The model under review builds one solid part; all positions refer to its coordinate system, in mm. A direction names the side the tool comes from. Coordinates: 2 decimals unless noted, no trailing zeros. Write each loop counter-clockwise with the first axis right and the second up, starting at its lowest first coordinate (ties: lowest second). Pieces come first, ordered by that corner, then holes. Notation, with made-up numbers: M 25,42 L 76,42 A10 cw 76,55 Z; hole C 33,78.5 d4. An arc over 180 degrees is marked long. Answer as CSV lines item,"result". Start each with the question number.
Autodesk Fusion 360 part; units mm, degrees
sketch "Skizze1" plane through (0, 0, 0) normal (0, 0, 1) x (1, 0, 0)
  line L0 (12.8, 3.8) -> (-12.8, 3.8)
  line L1 (-12.8, 3.8) -> (-12.8, -3.8)
  line L2 (-12.8, -3.8) -> (12.8, -3.8)
  line L3 (12.8, -3.8) -> (12.8, 3.8)
  line L4 (12.8, 3.8) -> (-12.8, -3.8) construction
  line L5 (-12.8, 3.8) -> (12.8, -3.8) construction
  line L6 (-15.6, 6.6) -> (-15.6, -6.6)
  line L7 (-15.6, -6.6) -> (15.6, -6.6)
  line L8 (15.6, -6.6) -> (15.6, 6.6)
  line L9 (15.6, 6.6) -> (-15.6, 6.6)
  line L10 (12.8, 1.5) -> (-12.8, 1.5)
  line L11 (-12.8, 1.5) -> (-12.8, -1.5)
  line L12 (-12.8, -1.5) -> (12.8, -1.5)
  line L13 (12.8, -1.5) -> (12.8, 1.5)
  line L14 (12.8, 1.5) -> (-12.8, -1.5) construction
  line L15 (-12.8, 1.5) -> (12.8, -1.5) construction
  circle A0 centre (20.6, 0) radius 1.6
  circle A1 centre (-20.6, 0) radius 1.6
  circle A2 centre (20.6, 0) radius 4
  circle A3 centre (-20.6, 0) radius 4
  line L16 (-20.6, 4) -> (-15.6, 4)
  line L17 (-20.6, -4) -> (-15.6, -4)
  line L18 (20.6, 4) -> (15.6, 4)
  line L19 (20.6, -4) -> (15.6, -4)
  dimension "d1" = 25.6
  dimension "d2" = 7.6
  dimension "d3" = 2.8
  dimension "d4" = 3
  dimension "d5" = 3.2
  dimension "d6" = 5
  dimension "d7" = 3.2
  dimension "d8" = 5
  dimension "d9" = 8
  dimension "d10" = 8
extrude "Extrusion1" add sketch "Skizze1" along normal blind 4 contours L0 L1 L3 L10 | L1 L2 L3 L12 | L6 L7 L8 L9 | L6 A3 L16 L17 | A3 | L8 A2 L18 L19 | A2
sketch "Skizze2" plane through (0, 0, 4) normal (0, 0, 1) x (-1, 0, 0)
  circle A0 centre (-20.6, 0) radius 1.6
  line L0 (-12.8, -1.5) -> (-12.8, 1.5)
  line L1 (-12.8, 1.5) -> (12.8, 1.5)
  line L2 (12.8, 1.5) -> (12.8, -1.5)
  line L3 (12.8, -1.5) -> (-12.8, -1.5)
  circle A1 centre (20.6, 0) radius 1.6
  line L4 (-20.6, -4) -> (-15.6, -4)
  line L5 (-15.6, -4) -> (-15.6, -6.6)
  line L6 (-15.6, -6.6) -> (15.6, -6.6)
  line L7 (15.6, -6.6) -> (15.6, -4)
  line L8 (15.6, -4) -> (20.6, -4)
  arc A2 (20.6, -4) -> (20.6, 4) centre (20.6, 0) ccw
  line L9 (20.6, 4) -> (15.6, 4)
  line L10 (15.6, 4) -> (15.6, 6.6)
  line L11 (15.6, 6.6) -> (-15.6, 6.6)
  line L12 (-15.6, 6.6) -> (-15.6, 4)
  line L13 (-15.6, 4) -> (-20.6, 4)
  arc A3 (-20.6, 4) -> (-20.6, -4) centre (-20.6, 0) ccw
  line L14 (-12.8, -3.8) -> (12.8, -3.8)
  line L15 (12.8, -3.8) -> (12.8, 3.8)
  line L16 (12.8, 3.8) -> (-12.8, 3.8)
  line L17 (-12.8, 3.8) -> (-12.8, -3.8)
extrude "Extrusion2" add sketch "Skizze2" along normal blind 13
fillet "Abrundung1" radius 2 4 edges at (12.8, 2.65, 4) (12.8, -2.65, 4) (-12.8, -2.65, 4) (-12.8, 2.65, 4)
fillet "Abrundung2" radius 2.5 4 edges at (-15.6, -6.6, 8.5) (15.6, -6.6, 8.5) (15.6, 6.6, 8.5) (-15.6, 6.6, 8.5)
sketch "Skizze3" plane through (0, -6.6, 0) normal (0, -1, 0) x (1, 0, 0)
  line L0 (13.1, 0) -> (13.1, 17)
  line L1 (13.1, 17) -> (-13.1, 17)
  line L2 (-13.1, 17) -> (-13.1, 0)
  line L3 (-13.1, 0) -> (13.1, 0)
  circle A0 centre (0, 10.5) radius 3
  line L4 (5.8778, 17) -> (5.8778, 4) construction
  point P0 (5.8778, 10.5)
  dimension "d19" = 6
extrude "Extrusion3" cut sketch "Skizze3" against normal up to surface (13.2 mm away) contours A0
1) To check wall thickness, follow line 1 (X direction, y = 0, z = 11.5); line 2 (Y direction, x = 6.5, z = 9); line 3 (Z direction, x = 0, y = 5.25). State the ranges of each line that lie inside material, in increasing order. Write a range as [from, to].
2) Take a section at B-B on x = 0. Give the boundary of the cut face in (y, z), and give its area (3 significant figures).
3) Clearance check with flat-ended pins moving along their axes: pin 1 Ø5 at (y, z) = (-4, 7.5) entering from +X; pin 2 Ø3 at (y, z) = (-2.5, 10) entering from +X; pin 3 Ø9.5 at (x, z) = (0, 10.5) entering from -Y; pin 4 Ø5.5 at (x, z) = (-17, 6) entering from +Y. State where each tip first meets the part, or that it passes through.
4) Mouldability with a two-part tool opening along X and no side actions: class faces 5 (the cylindrical face through (-12.23, 2.63, 4.6)), 6 (the cylindrical face through (-14.887, 5.848, 8.381)), 7 (the cylindrical face through (14.887, -5.848, 8.381)) as +X half, -X half, draft (parallel to the pull), parting line (faces both ways), or undercut.
5) Take a section at D-D on y = 0. Give the boundary of the cut face in (x, z), and give its area (3 significant figures).
6) Take a section at A-A on z = 10.5. Give the number of separate pieces and of enclosed holes in the cut face, and give its area (3 significant figures).
7) Take a section at C-C on x = -12. Give the boundary of the cut face in (y, z), and give its area (3 significant figures).
8) Tool access review of faces 1 (the flat face through (0, -4, 17)), 2 (the flat face through (12.8, 0, 10)), 3 (the flat face through (-18, 4, 8)), 4 (the flat face through (0, 1.5, 2)): name each direction out of +Z, -Z, +X, -X, +Y, -Y from which nothing blocks a thin tool from reaching the whole face with its end or side.
Results:
1,line 1,"x = [-24.6, -22.2], [-19, -12.8], [12.8, 19], [22.2, 24.6]"
1,line 2,"y = [-6.6, -3.8], [3.8, 6.6]"
1,line 3,"z = [0, 7.5], [13.5, 17]"
2,outline,"M -6.6,0 L -1.5,0 L -1.5,4 L -3.8,4 L -3.8,7.5 L -6.6,7.5 Z; M -6.6,13.5 L -3.8,13.5 L -3.8,17 L -6.6,17 Z; M 1.5,0 L 6.6,0 L 6.6,7.5 L 3.8,7.5 L 3.8,4 L 1.5,4 Z; M 3.8,13.5 L 6.6,13.5 L 6.6,17 L 3.8,17 Z"
2,area,"80.0 mm²"
3,pin 1,"stops at x = 24.31"
3,pin 2,"stops at x = 24.47"
3,pin 3,"stops at y = -6.6"
3,pin 4,"stops at y = 6.32"
4,face 5,"undercut"
4,face 6,"-X half"
4,face 7,"+X half"
5,outline,"M -24.6,0 L -22.2,0 L -22.2,17 L -24.6,17 Z; M -19,0 L -12.8,0 L -12.8,17 L -19,17 Z; M 12.8,0 L 19,0 L 19,17 L 12.8,17 Z; M 22.2,0 L 24.6,0 L 24.6,17 L 22.2,17 Z"
5,area,"292 mm²"
6,separate pieces,"2"
6,enclosed holes,"2"
6,area,"292 mm²"
7,outline,"M -6.6,0 L -1.5,0 L -1.5,4.4 L -3.8,4.4 L -3.8,17 L -6.6,17 Z; M 1.5,0 L 6.6,0 L 6.6,17 L 3.8,17 L 3.8,4.4 L 1.5,4.4 Z"
7,area,"115 mm²"
8,face 1,"+Z, +X, -X, +Y, -Y"
8,face 2,"+Z"
8,face 3,"+Z, -Z, -X, +Y"
8,face 4,"+Z, -Z"
